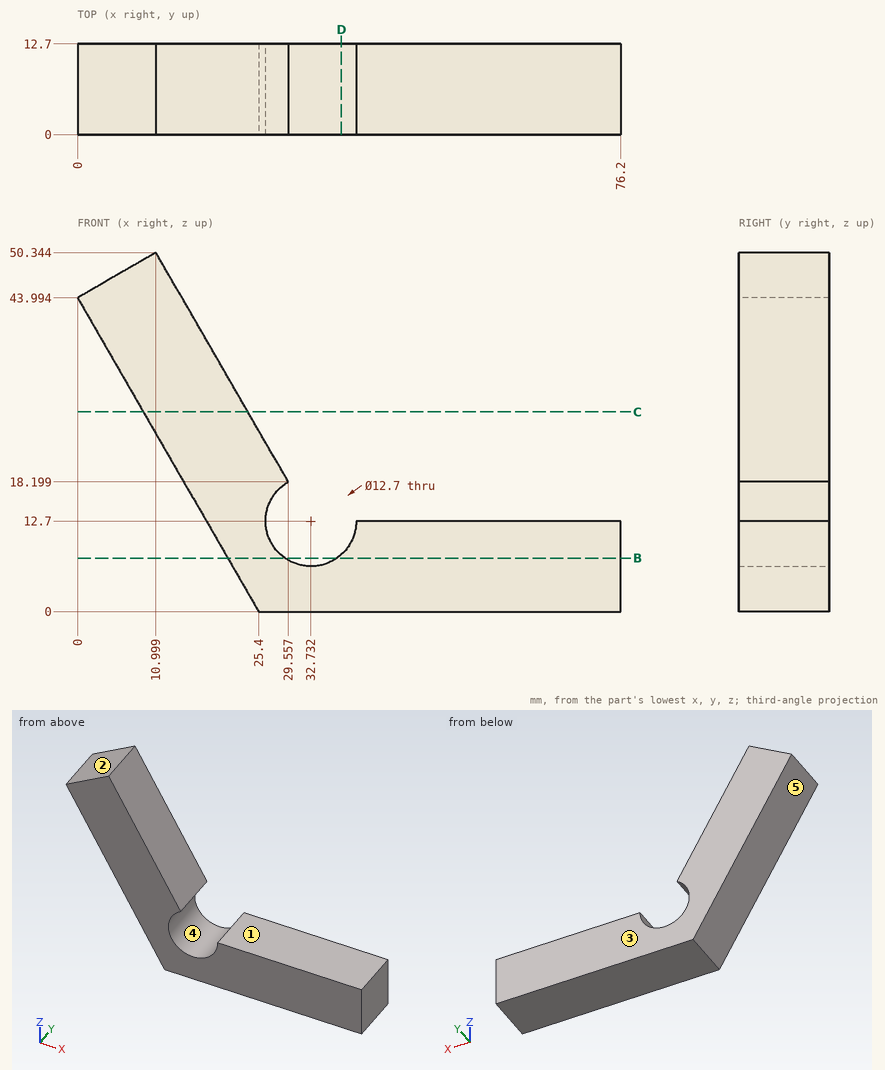
Part print with two shaded views. Sizes in mm from the minimum x, y, z corner. A direction names the side the tool comes from. Round coordinates to 2 decimals unless told otherwise and drop trailing zeros. Order: outer loops, then holes, each group sorted by start corner. A loop starts at its lowest first (then second) coordinate and runs counter-clockwise, first axis right, second up. Notation, with made-up numbers: M 54.25,86.25 L 92.25,86.25 A16 ccw 92.25,96.25 Z; hole C 68,25 d8. An arc over 180 degrees is marked long. Answer in a Markdown table with one row per item. Add a question column.
Q1. Mould opens along X. For the marked faces 3, 4 and 5 say: +X half, -X half, draft (parallel to the pull), parting line (faces both ways), or undercut.
Q2. Cut at D-D on x = 37. Give the cut face in (y, z).
Q3. Cut at B-B on z = 7.5. Give the cut face in (x, y).
Q4. Pin check, flat tips, straight feed: pin 1 (16.5 mm diameter, centred on x = 32.73, z = 12.7, fed in from +Y); pin 2 (1 mm diameter, centred on y = 3, z = 5.5, fed in from -X) (1 decimal). Stop position of each tip, or through.
Q5. Cut at C-C on z = 28. Give the cut face in (x, y) (1 decimal).
Q6. 3-axis set-ups, long thin cutter, end or side, ignore diameter. For the marked faces 1 and 2: which of +Z, -Z, +X, -X, +Y, -Y reach the whole face in a straight line?
Q7. Wall check: L1, parallel to Z at x = 46, y = 8.25; L2, parallel to X at y = 4.5, z = 8 (1 decimal); L3, parallel to Z at x = 33, y = 10 (1 decimal). Give the ranges that are in metal, low to high. Write a range as from..to.
Established:
| question | item | result |
|---|---|---|
| 1 | face 3 | draft |
| 1 | face 4 | undercut |
| 1 | face 5 | -X half |
| 2 | outline | M 0,0 L 12.7,0 L 12.7,8 L 0,8 Z |
| 3 | outline | M 21.07,0 L 29.09,0 L 29.09,12.7 L 21.07,12.7 Z; M 36.38,0 L 76.2,0 L 76.2,12.7 L 36.38,12.7 Z |
| 4 | pin 1 | stops at y = 12.7 |
| 4 | pin 2 | stops at x = 21.9 |
| 5 | outline | M 9.2,0 L 23.9,0 L 23.9,12.7 L 9.2,12.7 Z |
| 6 | face 1 | +Z, +X, +Y, -Y |
| 6 | face 2 | +Z, -X, +Y, -Y |
| 7 | L1 | z = 0..12.7 |
| 7 | L2 | x = 20.8..28.5, 37..76.2 |
| 7 | L3 | z = 0..6.4 |
